from build123d import *

# Parameters (mm, degrees)
SKETCH1_W           = 101.6
SKETCH1_H           = 60.96
BOSS_EXTRUDE1_DEPTH = 5.08
SKETCH2_W           = 96.52
SKETCH2_H           = 55.88
CUT_EXTRUDE1_DEPTH  = 3.81
SKETCH3_R           = 1.016
CUT_EXTRUDE3_DEPTH  = 11.43


with BuildPart() as part:
    # Sketch1 → Boss-Extrude1 (new body)
    with BuildSketch(Plane(origin=(-10.826110924, 0, 0), x_dir=(1, 0, 0), z_dir=(0, 1, 0))):
        with Locations((-6.069852941, -5.406838235)):
            Rectangle(SKETCH1_W, SKETCH1_H)
    extrude(amount=BOSS_EXTRUDE1_DEPTH)

    # Sketch2 → Cut-Extrude1 (cut)
    with BuildSketch(Plane(origin=(-10.826110924, 5.08, -21.022149646), x_dir=(1, 0, 0), z_dir=(0, 1, 0))):
        with Locations((-6.069852941, -26.428987881)):
            Rectangle(SKETCH2_W, SKETCH2_H)
    extrude(amount=-CUT_EXTRUDE1_DEPTH, mode=Mode.SUBTRACT)

    # Sketch3 → Cut-Extrude3 (cut)
    with BuildSketch(Plane(origin=(0, 1.27, -21.022149646), x_dir=(1, 0, 0), z_dir=(0, 1, 0))):
        with Locations((26.284036135, -3.568987881)):
            Circle(SKETCH3_R)
        with Locations((26.284036135, -49.288987881)):
            Circle(SKETCH3_R)
    extrude(amount=-CUT_EXTRUDE3_DEPTH, mode=Mode.SUBTRACT)


solid = part.part
Geometry check sheet. Reference: the model listing, model coordinates, mm. A direction names the side the tool comes from. Round coordinates to 2 decimals unless told otherwise and drop trailing zeros. Write each loop counter-clockwise with the first axis right and the second up, starting at its lowest first coordinate (ties: lowest second). Pieces come first, ordered by that corner, then holes. Notation, with made-up numbers: (-16, -4) -> (25, -4) arc R8 ccw to (25, 11) -> close; hole circle Ø9 at (30, 29). An arc over 180 degrees is marked (long way). One line per item, written item: value. Start each with the question number.
(1) Draft check along X on faces 1 (the flat face through (-18, 3, 33.347)), 2 (the flat face through (33.904, 3, 6)), 3 (the flat face through (-21, 5.08, 35)). Enter one of: +X half, -X half, draft (parallel to the pull), parting line (faces both ways), or undercut.
(2) Scan lines: line 1 (X direction, y = 4, z = -4.5); line 2 (Z direction, x = -4, y = 4.1); line 3 (Y direction, x = 17, z = -3). Record each from-to range of solid material in increasing order. Write a range as [from, to].
(3) Cross-section at A-A, the plane y = 2.35. Record the cut outline in (x, z).
(4) Cross-section at C-C, the plane z = -10. Record the cut outline in (x, y), and give its area (3 significant figures).
(5) Cross-section at B-B, the plane x = -50. Record the cut outline in (y, z), and give its area (3 significant figures).
(6) Access from +Z, -Z, +X, -X, +Y, -Y to the whole of each face (thin tool, end or side, straight path). Record for faces 4 (the flat face through (-18, 1.27, 5)), 5 (the cylindrical face through (25.27, 0.64, 28.22)).
(7) Go/stop test with a flat-tipped pin: pin 1 Ø17 at (x, z) = (-25.5, 2.5) entering from +Y. Record where the tip stops, or that it passes through.
Answer:
1. face 1: undercut
1. face 2: +X half
1. face 3: draft
2. line 1: [-67.7, -65.16], [31.36, 33.9]
2. line 2: [-25.07, -22.53], [33.35, 35.89]
2. line 3: [0, 1.27]
3. outline: (-67.7, -25.07) -> (33.9, -25.07) -> (33.9, 35.89) -> (-67.7, 35.89) -> close; hole (-65.16, -22.53) -> (31.36, -22.53) -> (31.36, 33.35) -> (-65.16, 33.35) -> close
4. outline: (-67.7, 0) -> (33.9, 0) -> (33.9, 5.08) -> (31.36, 5.08) -> (31.36, 1.27) -> (-65.16, 1.27) -> (-65.16, 5.08) -> (-67.7, 5.08) -> close
4. area: 148 mm²
5. outline: (0, -25.07) -> (5.08, -25.07) -> (5.08, -22.53) -> (1.27, -22.53) -> (1.27, 33.35) -> (5.08, 33.35) -> (5.08, 35.89) -> (0, 35.89) -> close
5. area: 96.8 mm²
6. face 4: +Y
6. face 5: +Y, -Y
7. pin 1: y = 1.27
